Design review of the part shown in the three views and the two pictorial views. Dimensions are in mm from the part's minimum x, y and z. Coordinates: 2 decimals unless noted, no trailing zeros. Write each loop counter-clockwise with the first axis right and the second up, starting at its lowest first coordinate (ties: lowest second). Pieces come first, ordered by that corner, then holes.
Q1. Take a section at B-B, the plane x = 64.5. Write out the cut boundary in (y, z) (3 decimals).
Q2. For pin 1 Ø1 at (y, z) = (2, 99.5) entering from +X (3 decimals); pin 2 Ø1.6 at (x, y) = (81.5, 2) entering from +Z, all flat-tipped, find the tip position at first contact; note any pin that passes through.
Q3. For L1, parallel to X at y = 2.05, z = 41 (3 decimals); L2, parallel to Z at x = 70, y = 0.6 (3 decimals), list the stretches that pass through material, from the lowest coordinate up.
Q4. Take a section at A-A, the plane z = 23. Write out the cut boundary in (x, y) (3 decimals).
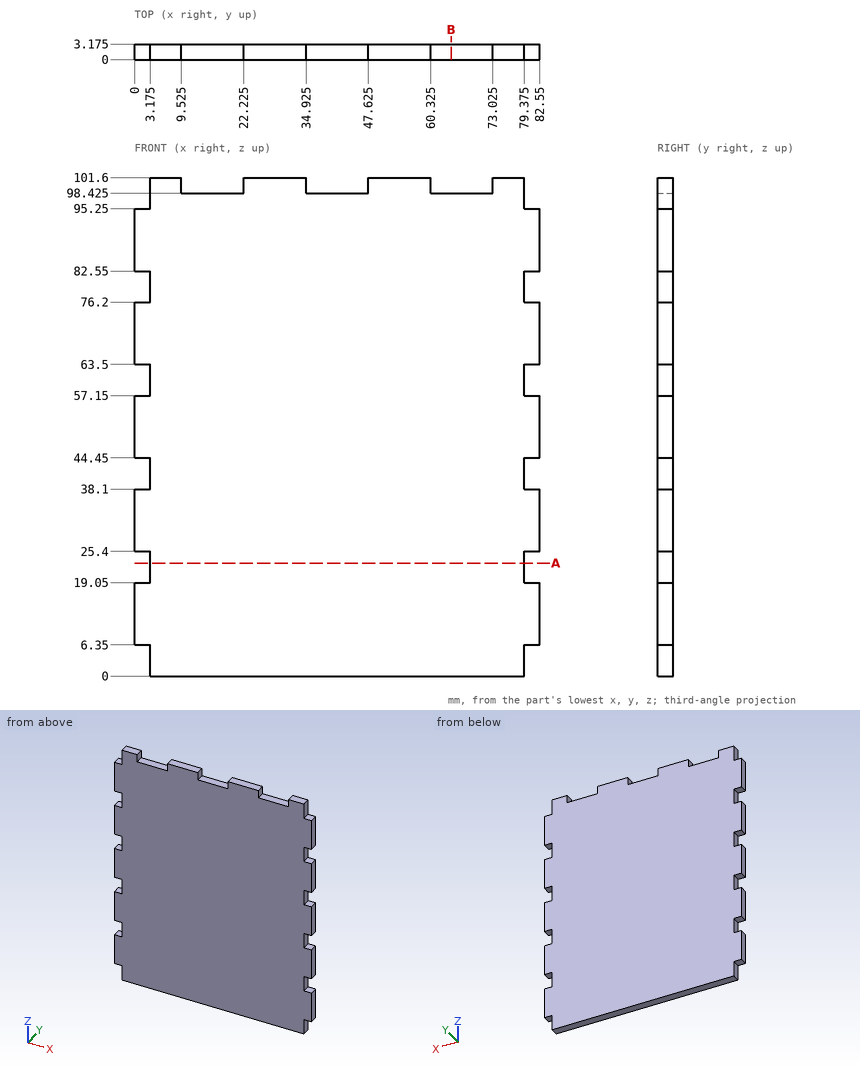
Responses:
1. outline: (0, 0) - (3.175, 0) - (3.175, 98.425) - (0, 98.425) - close
2. pin 1: stops at x = 79.375
2. pin 2: stops at z = 95.25
3. L1: x = 3.175 to 79.375
3. L2: z = 0 to 98.425
4. outline: (3.175, 0) - (79.375, 0) - (79.375, 3.175) - (3.175, 3.175) - close
